Model file for the job. Use its own axes, mm. A direction names the side the tool comes from. Give positions to 0.01 mm unless a question says otherwise; leave off trailing zeros. Write each loop counter-clockwise with the first axis right and the second up, starting at its lowest first coordinate (ties: lowest second). Pieces come first, ordered by that corner, then holes. Notation, with made-up numbers: (3.5, 88.25) - (53.5, 88.25) arc R18 ccw to (53.5, 94.25) - close; hole circle Ø7 at (66, 40.5). An arc over 180 degrees is marked (long way). Use CSV: the item, a comma, the result in double quotes.
Autodesk Inventor part; units mm, degrees
ref_plane "YZ Plane" through (0, 0, 0) normal (1, 0, 0) x (0, 1, 0)
ref_plane "XZ Plane" through (0, 0, 0) normal (0, 1, 0) x (-1, 0, 0)
ref_plane "XY Plane" through (0, 0, 0) normal (0, 0, 1) x (1, 0, 0)
sketch "Sketch1" plane through (0, 0, 0) normal (1, 0, 0) x (0, 1, 0)
  line L0 (0, 0) -> (50.8, 0)
  line L1 (50.8, 0) -> (50.8, -25.4)
  line L2 (50.8, -25.4) -> (0, -25.4)
  line L3 (0, -25.4) -> (0, 0)
  line L4 (49.53, -24.13) -> (49.53, -1.27)
  line L5 (49.53, -1.27) -> (1.27, -1.27)
  line L6 (1.27, -1.27) -> (1.27, -24.13)
  line L7 (1.27, -24.13) -> (49.53, -24.13)
  dimension "d0" = 50.8
  dimension "d1" = 25.4
  dimension "d2" = 1.27
extrude "Extrusion1" add sketch "Sketch1" along normal blind 609.6
sketch "Sketch2" plane through (0, 0, 0) normal (0, 0, 1) x (1, 0, 0)
  line L0 (537.5598, 19.0095) -> (541.0559, 18.8772)
  line L1 (534.0637, 19.1419) -> (537.5598, 19.0095)
  line L2 (532.1846, 22.3903) -> (533.818, 19.2964)
  arc A0 (533.818, 19.2964) -> (534.0637, 19.1419) centre (537.8, 25.355) ccw
  arc A1 (530.5621, 25.7742) -> (530.5512, 25.4841) centre (537.8, 25.355) ccw
  arc A2 (534.5441, 31.8328) -> (534.2874, 31.6973) centre (537.8, 25.355) ccw
  arc A3 (541.782, 31.4136) -> (541.5363, 31.5681) centre (537.8, 25.355) ccw
  arc A4 (545.0379, 24.9358) -> (545.0488, 25.2259) centre (537.8, 25.355) ccw
  arc A5 (541.0559, 18.8772) -> (541.3126, 19.0127) centre (537.8, 25.355) ccw
  circle A6 centre (537.8, 25.355) radius 7.25
  point P0 (0, 0)
extrude "Extrusion2" cut sketch "Sketch2" against normal through all
sketch "Sketch4" plane through (0, 0, 0) normal (0, 0, 1) x (1, 0, 0)
  circle A0 centre (352.9118, 25.4) radius 7.3323
  circle A1 centre (174.2245, 25.4) radius 7.3323
  point P0 (0, 0)
extrude "Extrusion4" cut sketch "Sketch4" against normal through all
sketch "Sketch5" plane through (0, 0, -25.4) normal (0, 0, -1) x (-1, 0, 0)
  line L0 (0, 50.8) -> (-609.6, 50.8)
  line L1 (0, 50.8) -> (-15.2407, 0)
  line L2 (0, 0) -> (-609.6, 0)
  line L3 (0, 50.8) -> (53.037, 50.8) construction
  line L4 (0, 50.8) -> (0, 0)
  line L5 (0, 0) -> (-15.2407, 0)
  line L6 (0, 1.27) -> (-609.6, 1.27)
  dimension "d12" = 106.7
extrude "Extrusion5" cut sketch "Sketch5" against normal blind 25.4
properties part number "Aluminum Channel Arm Left"
(1) Pull direction X, two halves, no side cores. Call faces 1 (the face through (609.6, 23, -25)), 2 (the face through (181.22, 27.6, -24.76)), 3 (the face through (308, 1.27, -13)): released by +X, released by -X, zero draft, split by the parting line, or undercut.
Checked values:
face 1,"released by +X"
face 2,"undercut"
face 3,"zero draft"
(2) Flat gauge pin, fed straight in: P1, Ø19, axis at x = 174.22, y = 25.4, coming from the -Z side. Where does the tip first touch, or does it go through?
Checked values:
P1,"stops at z = -25.4"
(3) 3-axis set-ups, long thin cutter, end or side, ignore diameter. For faces 4 (the face through (7.02, 27.4, -0.53)), 5 (the face through (301, 26, -1.27)): which of +Z, -Z, +X, -X, +Y, -Y reach the whole face in a straight line?
Checked values:
face 4,"+Z, -Z, -X, -Y"
face 5,"+X, -X"
(4) Saw through at B-B, the plane x = 212.5. List the corners of the cut face in (y, z), then the cut area to 3 significant figures.
Checked values:
outline,"(0, -25.4) - (50.8, -25.4) - (50.8, 0) - (0, 0) - close; hole (1.27, -24.13) - (49.53, -24.13) - (49.53, -1.27) - (1.27, -1.27) - close"
area,"187 mm^2"
(5) Saw through at A-A, the plane z = -19. List the corners of the cut face in (x, y), then the cut area to 3 significant figures.
Checked values:
outline,"(0, 50.8) - (0.38, 49.53) - (609.6, 49.53) - (609.6, 50.8) - close; (14.86, 1.27) - (15.24, 0) - (609.6, 0) - (609.6, 1.27) - close"
area,"1,530 mm^2"
(6) Wall check: probe 1 along Z at (x, y) = (557, 20.5); probe 2 along Y at (x, z) = (133, -19.75). Give the ranges that are in metal, low to high. Write a range as [from, to].
Checked values:
probe 1,"z = [-25.4, -24.13], [-1.27, 0]"
probe 2,"y = [0, 1.27], [49.53, 50.8]"
